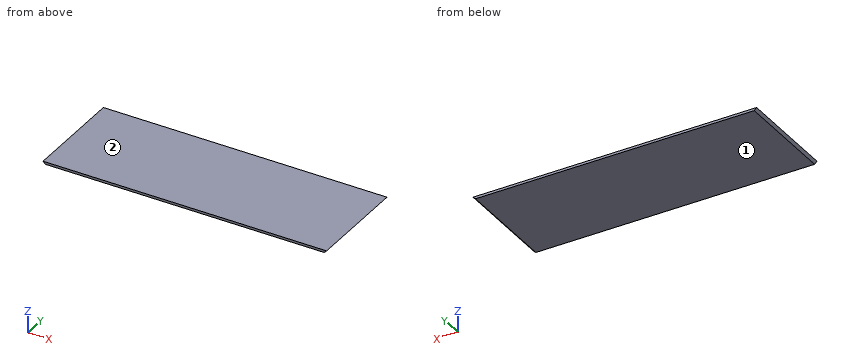
```python
from build123d import *

# Parameters (mm, degrees)
F0_W     = 2133.6
F0_H     = 762
F1_DEPTH = 17.99844
F2_SIZE  = 17.99843


# Not quite as in the source:
# - a fillet or chamfer is up to 0.001 mm smaller than in the source, because OpenCascade refuses the exact size


with BuildPart() as f1:
    # F0 (on Top) → F1 (new body)
    with BuildSketch(Plane.XY):
        with Locations((1066.8, 381)):
            Rectangle(F0_W, F0_H)
    extrude(amount=-F1_DEPTH)

    # F2 (size 17.99844 in the source; OpenCascade refuses exactly that, so slightly less here)
    f2_edges = [f1.edges().sort_by_distance(p)[0] for p in [
        (2133.6, 381, -17.99844),
        (0, 381, -17.99844),
    ]]
    chamfer(f2_edges, length=F2_SIZE)


solid = f1.part
```
Geometry check sheet. Reference: the model listing, model coordinates, mm. Face numbers are marked on the shaded views. Coordinates: 2 decimals unless noted, no trailing zeros.
Item 1: Mould release check, pull along Z, two halves, no side actions. Record for the marked faces 1 and 2: released by +Z, released by -Z, zero draft, split by the parting line, or undercut.
Item 2: Scan lines: line 1 along X through (y, z) = (490, -4.5); line 2 along X through (y, z) = (593.5, -3). Record each from-to range of solid material in increasing order.
Item 3: Depth check by flat-ended pin: pin 1 (2 mm diameter, centred on y = 413, z = -5, fed in from +X); pin 2 (5 mm diameter, centred on y = 242, z = -12.5, fed in from -X). Enter the tip coordinate at first touch or a pass-through.
Check sheet entries:
1. face 1: released by -Z
1. face 2: released by +Z
2. line 1: x = 4.5 to 2129.1
2. line 2: x = 3 to 2130.6
3. pin 1: stops at x = 2129.6
3. pin 2: stops at x = 10
